For this review, take the finished solid that the model builds, in its own axes (mm). Face numbers are marked on the shaded views. A direction names the side the tool comes from. Coordinates: 2 decimals unless noted, no trailing zeros. Loops run counter-clockwise (first coordinate to the right, second up) from the corner with the lowest first, then second, coordinate; pieces in that order, holes last.
1. Machinability: for the marked faces 4, 5 and 6, which of the approach directions +Z, -Z, +X, -X, +Y, -Y give a long, thin tool a straight path to every point of the face, cutting with its end or side? Answer none if there is none.
2. Take a section at D-D, the plane x = 0. State the section outline as (y, z) points.
3. Mouldability with a two-part tool opening along Y and no side actions: class the marked faces 1, 2 and 3 as pulls with the +Y half, pulls with the -Y half, needs draft (parallel to the pull), parting line crosses it, or undercut.
4. Clearance check with flat-ended pins moving along their axes: P1, Ø1.2, axis at x = 12, z = 1, coming from the +Y side; P2, Ø1, axis at y = 4, z = 2, coming from the -X side. State where each tip first meets the part, or that it passes through.
5. To check wall thickness, follow probe 1 along X at (y, z) = (-11, 1.85); probe 2 along Y at (x, z) = (-12, 2.95); probe 3 along X at (y, z) = (-0.5, 3). State the ranges of each line that lie inside material, in increasing order.
6. Take a section at C-C, the plane y = -11. State the section outline as (x, z) points.
7. Take a section at B-B, the plane x = -12. State the section outline as (y, z) points.
8. Take a section at A-A, the plane z = 2.65. State the section outline as (x, y) points.
```python
from build123d import *

# Parameters (mm, degrees)
F0_W     = 12
F0_H     = 8
F1_DEPTH = 4
F2_D     = 2.7
F3_R     = 6
F4_R     = 2


with BuildPart() as f1:
    # F0 (on Top) → F1 (new body)
    with BuildSketch(Plane.XY):
        Polygon((-4, -15), (4, -15), (4, -7), (4, 15), (-4, 15), (-4, -7), align=None)
        with Locations((10, -11)):
            Rectangle(F0_W, F0_H)
        with Locations((-10, -11)):
            Rectangle(F0_W, F0_H)
    extrude(amount=F1_DEPTH)

    # F2 (through all)
    with Locations(Plane(origin=(0, 0, 0), x_dir=(1, 0, 0), z_dir=(0, 0, -1))):
        with Locations((0, -11), (12, 11), (0, 0), (-12, 11), (0, -10.5), (0, -11.5), (0, -0.5), (0, 0.5)):
            Hole(F2_D / 2)

    # F3
    f3_edges = [f1.edges().sort_by_distance(p)[0] for p in [
        (-4, -7, 2),
        (4, -7, 2),
    ]]
    fillet(f3_edges, radius=F3_R)

    # F4
    f4_edges = [f1.edges().sort_by_distance(p)[0] for p in [
        (-4, 15, 2),
        (4, 15, 2),
        (16, -7, 2),
        (16, -15, 2),
        (-16, -7, 2),
        (-16, -15, 2),
    ]]
    fillet(f4_edges, radius=F4_R)


solid = f1.part
```
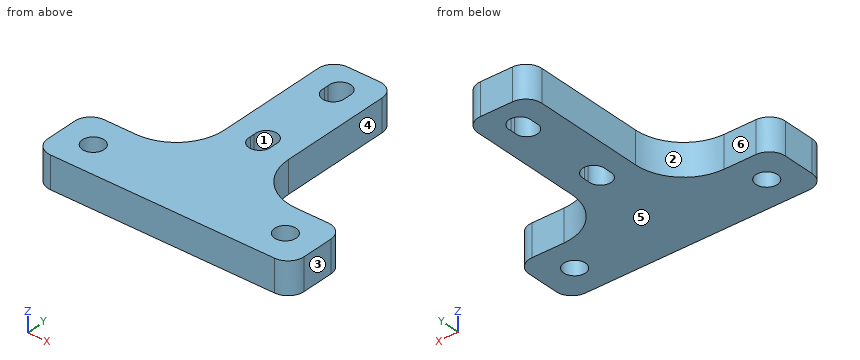
Results list:
1. face 4: +Z, -Z, +X, +Y
1. face 5: -Z, +X, -X, +Y, -Y
1. face 6: +Z, -Z, -X, +Y
2. outline: (-15, 0) - (-1.85, 0) - (-1.85, 4) - (-15, 4) - close; (1.85, 0) - (9.15, 0) - (9.15, 4) - (1.85, 4) - close; (12.85, 0) - (15, 0) - (15, 4) - (12.85, 4) - close
3. face 1: undercut
3. face 2: pulls with the +Y half
3. face 3: needs draft
4. P1: stops at y = -7
4. P2: stops at x = -4
5. probe 1: x = -16 to -13.35, -10.65 to 10.65, 13.35 to 16
5. probe 2: y = -15 to -12.35, -9.65 to -7
5. probe 3: x = -4 to -1.35, 1.35 to 4
6. outline: (-16, 0) - (-13.35, 0) - (-13.35, 4) - (-16, 4) - close; (-10.65, 0) - (10.65, 0) - (10.65, 4) - (-10.65, 4) - close; (13.35, 0) - (16, 0) - (16, 4) - (13.35, 4) - close
7. outline: (-15, 0) - (-12.35, 0) - (-12.35, 4) - (-15, 4) - close; (-9.65, 0) - (-7, 0) - (-7, 4) - (-9.65, 4) - close
8. outline: (-16, -13) arc R2 ccw to (-14, -15) - (14, -15) arc R2 ccw to (16, -13) - (16, -9) arc R2 ccw to (14, -7) - (10, -7) arc R6 cw to (4, -1) - (4, 13) arc R2 ccw to (2, 15) - (-2, 15) arc R2 ccw to (-4, 13) - (-4, -1) arc R6 cw to (-10, -7) - (-14, -7) arc R2 ccw to (-16, -9) - close; hole circle Ø2.7 at (-12, -11); hole (-1.33, -0.25) arc R1.35 ccw (long way) to (1.33, -0.25) arc R1.35 ccw to (1.33, 0.25) arc R1.35 ccw (long way) to (-1.33, 0.25) arc R1.35 ccw to start; hole (-1.33, 10.75) arc R1.35 ccw (long way) to (1.33, 10.75) arc R1.35 ccw to (1.33, 11.25) arc R1.35 ccw (long way) to (-1.33, 11.25) arc R1.35 ccw to start; hole circle Ø2.7 at (12, -11)
